from build123d import *

# Parameters (mm, degrees)
SKETCH2_R           = 14
BOSS_EXTRUDE1_DEPTH = 24
SKETCH3_R           = 3.95
BOSS_EXTRUDE2_DEPTH = 7
SKETCH4_R           = 3
BOSS_EXTRUDE3_DEPTH = 7
SKETCH6_R           = 1.5
CUT_EXTRUDE1_DEPTH  = 5


with BuildPart() as part:
    # Sketch2 → Boss-Extrude1 (new body)
    with BuildSketch(Plane(origin=(0, 0, 0), x_dir=(1, 0, 0), z_dir=(0, 1, 0))):
        with Locations(Location((0, 0, 0), (0, 0, 270))):
            Circle(SKETCH2_R)
    extrude(amount=BOSS_EXTRUDE1_DEPTH)

    # Sketch3 → Boss-Extrude2 (add)
    with BuildSketch(Plane(origin=(0, 24, 0), x_dir=(1, 0, 0), z_dir=(0, 1, 0))):
        with Locations(Location((0, 0, 0), (0, 0, 270))):
            Circle(SKETCH3_R)
    extrude(amount=BOSS_EXTRUDE2_DEPTH)

    # Sketch4 → Boss-Extrude3 (add)
    with BuildSketch(Plane(origin=(0, 31, 0), x_dir=(1, 0, 0), z_dir=(0, 1, 0))):
        with Locations(Location((0, 0, 0), (0, 0, 270))):
            Circle(SKETCH4_R)
    extrude(amount=BOSS_EXTRUDE3_DEPTH)

    # Sketch6 → Cut-Extrude1 (cut)
    with BuildSketch(Plane.XZ):
        with Locations(Location((9.5, 0, 0), (0, 0, 270))):
            Circle(SKETCH6_R)
        with Locations(Location((0, -9.5, 0), (0, 0, 270))):
            Circle(SKETCH6_R)
        with Locations(Location((-9.5, 0, 0), (0, 0, 270))):
            Circle(SKETCH6_R)
        with Locations(Location((0, 9.5, 0), (0, 0, 270))):
            Circle(SKETCH6_R)
    extrude(amount=-CUT_EXTRUDE1_DEPTH, mode=Mode.SUBTRACT)


solid = part.part
Verification items for the finished model (mm, model axes). A direction names the side the tool comes from. Give positions to 0.01 mm unless a question says otherwise; leave off trailing zeros. Write each loop counter-clockwise with the first axis right and the second up, starting at its lowest first coordinate (ties: lowest second). Pieces come first, ordered by that corner, then holes. Notation, with made-up numbers: (81.25, 69) - (98.25, 69) arc R9 ccw to (98.25, 83) - close; hole circle Ø9 at (-12.75, 42.25). An arc over 180 degrees is marked (long way). Answer as CSV lines item,"result". Start each with the question number.
1. Thickness scan on line 1 (X direction, y = 3.6, z = 0); line 2 (Y direction, x = -2.5, z = 4.5); line 3 (X direction, y = 2.7, z = 9.5). Record the ranges inside material, lowest first.
2. Sectioned sample at B-B (x = 0). Record the boundary of the cut face in (y, z).
3. Sectioned sample at D-D (x = 8.5). Record the boundary of the cut face in (y, z), then the cut area to 3 significant figures.
4. Draft check along X on faces 4 (the face through (-9, 5, 0)), 5 (the face through (0, 5, 10)), 6 (the face through (0.9, 34.45, 2.86)), 7 (the face through (-3, 24, 3)). Enter one of: pulls with the +X half, pulls with the -X half, needs draft (parallel to the pull), parting line crosses it, or undercut.
5. Depth check by flat-ended pin: pin 1 (2.5 mm diameter, centred on x = 0, z = -9.5, fed in from -Y); pin 2 (2 mm diameter, centred on x = -5, y = 14, fed in from +Z); pin 3 (3 mm diameter, centred on y = 20.5, z = -10, fed in from -X). Enter the tip coordinate at first touch or a pass-through.
6. Sectioned sample at C-C (y = 36.5). Record the boundary of the cut face in (x, z), then the cut area to 3 significant figures.
7. Sectioned sample at A-A (z = 0). Record the boundary of the cut face in (x, y), then the cut area to 3 significant figures.
8. Set-up check for faces 1 (the face through (2.67, 27.45, -2.91)), 2 (the face through (-13.67, 11.83, -3.03)), 3 (the face through (10, 5, 0)): record each of +Z, -Z, +X, -X, +Y, -Y from which the full face is reachable in a straight line by a thin tool's end or side.
Derived:
1,line 1,"-14 to -11, -8 to 8, 11 to 14"
1,line 2,"0 to 24"
1,line 3,"-10.28 to -1.5, 1.5 to 10.28"
2,outline,"(0, -14) - (24, -14) - (24, -3.95) - (31, -3.95) - (31, -3) - (38, -3) - (38, 3) - (31, 3) - (31, 3.95) - (24, 3.95) - (24, 14) - (0, 14) - (0, 11) - (5, 11) - (5, 8) - (0, 8) - (0, -8) - (5, -8) - (5, -11) - (0, -11) - close"
3,outline,"(0, -11.12) - (24, -11.12) - (24, 11.12) - (0, 11.12) - (0, 1.12) - (5, 1.12) - (5, -1.12) - (0, -1.12) - close"
3,area,"523 mm²"
4,face 4,"undercut"
4,face 5,"undercut"
4,face 6,"parting line crosses it"
4,face 7,"needs draft"
5,pin 1,"y = 5"
5,pin 2,"z = 13.42"
5,pin 3,"x = -11.12"
6,outline,"circle Ø6 at (0, 0)"
6,area,"28.3 mm²"
7,outline,"(-14, 0) - (-11, 0) - (-11, 5) - (-8, 5) - (-8, 0) - (8, 0) - (8, 5) - (11, 5) - (11, 0) - (14, 0) - (14, 24) - (3.95, 24) - (3.95, 31) - (3, 31) - (3, 38) - (-3, 38) - (-3, 31) - (-3.95, 31) - (-3.95, 24) - (-14, 24) - close"
7,area,"739 mm²"
8,face 1,"+Y"
8,face 2,"+Y, -Y"
8,face 3,"-Y"
